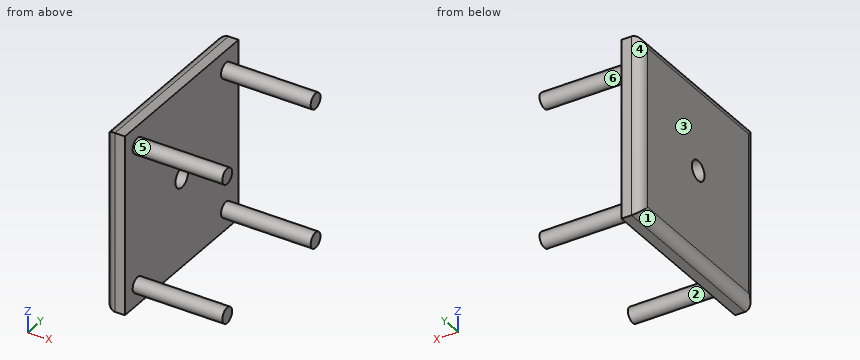
```python
from build123d import *

# Parameters (mm, degrees)
SKETCH1_W           = 18
SKETCH1_H           = 18
SKETCH1_R           = 0.75
BOSS_EXTRUDE1_DEPTH = 2
SKETCH2_R           = 0.775
BOSS_EXTRUDE2_DEPTH = 9
SKETCH3_R           = 1
CUT_EXTRUDE1_DEPTH  = 9
FILLET2_R           = 1


with BuildPart() as part:
    # Sketch1 → Boss-Extrude1 (new body)
    # profile 1 of 5: a face of its own
    with BuildSketch(Plane(origin=(0, 0, 0), x_dir=(0, 0, -1), z_dir=(1, 0, 0))):
        Rectangle(SKETCH1_W, SKETCH1_H)
        with Locations((-7, -7)):
            Circle(SKETCH1_R, mode=Mode.SUBTRACT)
        with Locations((7, -7)):
            Circle(SKETCH1_R, mode=Mode.SUBTRACT)
        with Locations((7, 7)):
            Circle(SKETCH1_R, mode=Mode.SUBTRACT)
        with Locations((-7, 7)):
            Circle(SKETCH1_R, mode=Mode.SUBTRACT)
    # profile 2 of 5: a face of its own
    with BuildSketch(Plane(origin=(0, 0, 0), x_dir=(0, 0, -1), z_dir=(1, 0, 0))):
        with Locations((7, 7)):
            Circle(SKETCH1_R)
    # profile 3 of 5: a face of its own
    with BuildSketch(Plane(origin=(0, 0, 0), x_dir=(0, 0, -1), z_dir=(1, 0, 0))):
        with Locations((-7, 7)):
            Circle(SKETCH1_R)
    # profile 4 of 5: a face of its own
    with BuildSketch(Plane(origin=(0, 0, 0), x_dir=(0, 0, -1), z_dir=(1, 0, 0))):
        with Locations((-7, -7)):
            Circle(SKETCH1_R)
    # profile 5 of 5: a face of its own
    with BuildSketch(Plane(origin=(0, 0, 0), x_dir=(0, 0, -1), z_dir=(1, 0, 0))):
        with Locations((7, -7)):
            Circle(SKETCH1_R)
    extrude(amount=BOSS_EXTRUDE1_DEPTH)

    # Sketch2 → Boss-Extrude2 (add)
    with BuildSketch(Plane(origin=(2, 0, 0), x_dir=(0, 0, -1), z_dir=(1, 0, 0))):
        with Locations((-7, 7)):
            Circle(SKETCH2_R)
        with Locations((-7, -7)):
            Circle(SKETCH2_R)
        with Locations((7, -7)):
            Circle(SKETCH2_R)
        with Locations((7, 7)):
            Circle(SKETCH2_R)
    extrude(amount=BOSS_EXTRUDE2_DEPTH)

    # Sketch3 → Cut-Extrude1 (cut)
    with BuildSketch(Plane.ZY):
        Circle(SKETCH3_R)
    extrude(amount=-CUT_EXTRUDE1_DEPTH, mode=Mode.SUBTRACT)

    # Fillet2
    fillet2_edges = [part.edges().sort_by_distance(p)[0] for p in [
        (0, 0, 9),
        (0, 9, 0),
        (0, 0, -9),
        (0, -9, 0),
    ]]
    fillet(fillet2_edges, radius=FILLET2_R)


solid = part.part
```
Can you work these out from the model? Positions are in its coordinate system, mm. Face numbers are marked on the shaded views. A direction names the side the tool comes from. Coordinates: 2 decimals unless noted, no trailing zeros. Order: outer loops, then holes, each group sorted by start corner. A loop starts at its lowest first (then second) coordinate and runs counter-clockwise, first axis right, second up.
1. I need wall thicknesses on line 1 (Y direction, x = 1.2, z = 0); line 2 (Y direction, x = 2.75, z = 7) (3 decimals); line 3 (X direction, y = -4.75, z = -2.75). Which ranges of each line are inside material? Lowest first, please.
2. If we section it at A-A (y = 0): Please give me the cut outline in (x, z).
3. For the marked faces 1 and 2, which set-ups out of +Z, -Z, +X, -X, +Y, -Y let a thin tool reach every point of the face, with its end or its side?
4. If we section it at C-C (z = -7): Please give me the cut outline in (x, y) (3 decimals).
5. Thinking about a two-plate mould opening in Y: for the marked faces 3, 4, 5 and 6, which applies, +Y half, -Y half, draft (parallel to the pull), parting line (faces both ways), or undercut?
6. I'm going to push flat-ended pins straight in: pin 1 (5 mm diameter, centred on y = -2, z = 2.5, fed in from +X); pin 2 (2 mm diameter, centred on x = 5, y = 6.5, fed in from -Z) (3 decimals). Where does each tip first touch, or does it pass through?
Entries:
1. line 1: y = -9 to -1, 1 to 9
1. line 2: y = -7.775 to -6.225, 6.225 to 7.775
1. line 3: x = 0 to 2
2. outline: (0, -8) arc R1 ccw to (1, -9) - (2, -9) - (2, -1) - (0, -1) - close; (0, 1) - (2, 1) - (2, 9) - (1, 9) arc R1 ccw to (0, 8) - close
3. face 1: -Z, -X, +Y, -Y
3. face 2: +X
4. outline: (0, -8) arc R1 ccw to (1, -9) - (2, -9) - (2, -7.775) - (11, -7.775) - (11, -6.225) - (2, -6.225) - (2, 6.225) - (11, 6.225) - (11, 7.775) - (2, 7.775) - (2, 9) - (1, 9) arc R1 ccw to (0, 8) - close
5. face 3: draft
5. face 4: +Y half
5. face 5: undercut
5. face 6: undercut
6. pin 1: stops at x = 2
6. pin 2: stops at z = -7.775
